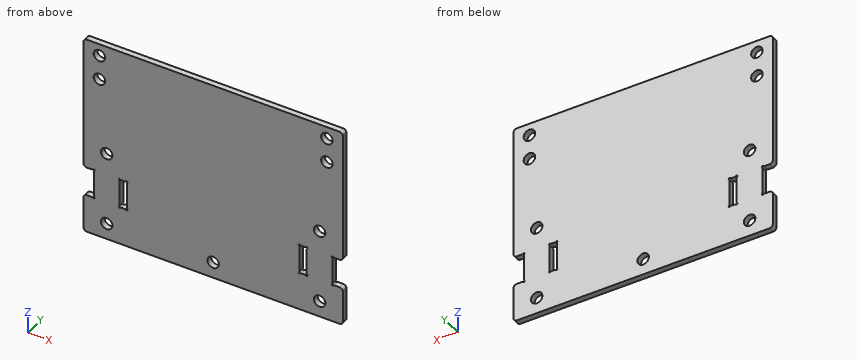
from build123d import *

# Parameters (mm, degrees)
STOCK_BEE_ZERKER_START                     = 4.064
STOCK_BEE_ZERKER_2_0_MULTIBODY_1_OUTLINE_R = 2.2479
STOCK_BEE_ZERKER_2_0_MULTIBODY_1_OUTLINE_W = 2.54
STOCK_BEE_ZERKER_2_0_MULTIBODY_1_OUTLINE_H = 10.89526775
STOCK_BEE_ZERKER_2_0_MULTIBODY_1_DEPTH     = 2.286
SKETCH1_W                                  = 2.794
SKETCH1_H                                  = 11.14926775
SKETCH1_W_2                                = 2.54
SKETCH1_H_2                                = 10.89526775
CUT_EXTRUDE1_DEPTH                         = 67.506087708
SKETCH2_R                                  = 0.3175
CUT_EXTRUDE2_DEPTH                         = 67.327231853
FILLET1_R                                  = 0.635
FILLET2_R                                  = 1.27


# Read off the part's stored shape, not the designer's step: Stock-Bee-zerker 2.0 Multibody-1
with BuildPart() as part:
    # Stock-Bee-zerker 2.0 Multibody-1 outline → Stock-Bee-zerker 2.0 Multibody-1 (new body)
    with BuildSketch(Plane(origin=(0, 0, 0), x_dir=(1, 0, 0), z_dir=(0, 1, 0)).offset(STOCK_BEE_ZERKER_START)):
        Polygon((-50.8, 16.917066125), (-50.8, -35.16122), (50.8, -35.16122), (50.8, 16.917066125), (46.7868, 16.917066125), (46.7868, 27.812333875), (50.8, 27.812333875), (50.8, 42.8625), (-50.8, 42.8625), (-50.8, 27.812333875), (-46.7868, 27.812333875), (-46.7868, 16.917066125), align=None)
        with Locations((-44.45, -30.39872)):
            Circle(STOCK_BEE_ZERKER_2_0_MULTIBODY_1_OUTLINE_R, mode=Mode.SUBTRACT)
        with Locations((-44.45, -20.87372)):
            Circle(STOCK_BEE_ZERKER_2_0_MULTIBODY_1_OUTLINE_R, mode=Mode.SUBTRACT)
        with Locations((44.45, -30.39872)):
            Circle(STOCK_BEE_ZERKER_2_0_MULTIBODY_1_OUTLINE_R, mode=Mode.SUBTRACT)
        with Locations((44.45, -20.87372)):
            Circle(STOCK_BEE_ZERKER_2_0_MULTIBODY_1_OUTLINE_R, mode=Mode.SUBTRACT)
        with Locations((-41.6052, 8.2169)):
            Circle(STOCK_BEE_ZERKER_2_0_MULTIBODY_1_OUTLINE_R, mode=Mode.SUBTRACT)
        with Locations((-35.1536, 22.3647)):
            Rectangle(STOCK_BEE_ZERKER_2_0_MULTIBODY_1_OUTLINE_W, STOCK_BEE_ZERKER_2_0_MULTIBODY_1_OUTLINE_H, mode=Mode.SUBTRACT)
        with Locations((-41.6052, 36.5125)):
            Circle(STOCK_BEE_ZERKER_2_0_MULTIBODY_1_OUTLINE_R, mode=Mode.SUBTRACT)
        with Locations((0, 36.5125)):
            Circle(STOCK_BEE_ZERKER_2_0_MULTIBODY_1_OUTLINE_R, mode=Mode.SUBTRACT)
        with Locations((41.6052, 8.2169)):
            Circle(STOCK_BEE_ZERKER_2_0_MULTIBODY_1_OUTLINE_R, mode=Mode.SUBTRACT)
        with Locations((35.1536, 22.3647)):
            Rectangle(STOCK_BEE_ZERKER_2_0_MULTIBODY_1_OUTLINE_W, STOCK_BEE_ZERKER_2_0_MULTIBODY_1_OUTLINE_H, mode=Mode.SUBTRACT)
        with Locations((41.6052, 36.5125)):
            Circle(STOCK_BEE_ZERKER_2_0_MULTIBODY_1_OUTLINE_R, mode=Mode.SUBTRACT)
    extrude(amount=STOCK_BEE_ZERKER_2_0_MULTIBODY_1_DEPTH)

    # Sketch1 → Cut-Extrude1 (cut, through all)
    # profile 1 of 3: a face of its own
    with BuildSketch(Plane(origin=(0, 6.35, 0), x_dir=(1, 0, 0), z_dir=(0, 1, 0))):
        Polygon((-46.7868, 16.917066125), (-50.8, 16.917066125), (-50.8, -35.16122), (50.8, -35.16122), (50.8, 16.917066125), (46.7868, 16.917066125), (46.7868, 27.812333875), (50.8, 27.812333875), (50.8, 42.8625), (-50.8, 42.8625), (-50.8, 27.812333875), (-46.7868, 27.812333875), align=None)
        Polygon((-46.6598, 16.790066125), (-50.673, 16.790066125), (-50.673, -35.03422), (50.673, -35.03422), (50.673, 16.790066125), (46.6598, 16.790066125), (46.6598, 27.939333875), (50.673, 27.939333875), (50.673, 42.7355), (-50.673, 42.7355), (-50.673, 27.939333875), (-46.6598, 27.939333875), align=None, mode=Mode.SUBTRACT)
    # profile 2 of 3: a face of its own
    with BuildSketch(Plane(origin=(0, 6.35, 0), x_dir=(1, 0, 0), z_dir=(0, 1, 0))):
        with Locations((-35.1536, 22.3647)):
            Rectangle(SKETCH1_W, SKETCH1_H)
        with Locations((-35.1536, 22.3647)):
            Rectangle(SKETCH1_W_2, SKETCH1_H_2, mode=Mode.SUBTRACT)
    # profile 3 of 3: a face of its own
    with BuildSketch(Plane(origin=(0, 6.35, 0), x_dir=(1, 0, 0), z_dir=(0, 1, 0))):
        with Locations((35.1536, 22.3647)):
            Rectangle(SKETCH1_W, SKETCH1_H)
        with Locations((35.1536, 22.3647)):
            Rectangle(SKETCH1_W_2, SKETCH1_H_2, mode=Mode.SUBTRACT)
    extrude(amount=-CUT_EXTRUDE1_DEPTH, mode=Mode.SUBTRACT)

    # Sketch2 → Cut-Extrude2 (cut, through all)
    with BuildSketch(Plane(origin=(0, 6.35, 0), x_dir=(1, 0, 0), z_dir=(0, 1, 0))):
        with Locations((-46.6598, 27.939333875)):
            Circle(SKETCH2_R)
        with Locations((-46.6598, 16.790066125)):
            Circle(SKETCH2_R)
        with Locations((-36.5506, 16.790066125)):
            Circle(SKETCH2_R)
        with Locations((-33.7566, 16.790066125)):
            Circle(SKETCH2_R)
        with Locations((-33.7566, 27.939333875)):
            Circle(SKETCH2_R)
        with Locations((-36.5506, 27.939333875)):
            Circle(SKETCH2_R)
        with Locations((33.7566, 27.939333875)):
            Circle(SKETCH2_R)
        with Locations((36.5506, 27.939333875)):
            Circle(SKETCH2_R)
        with Locations((33.7566, 16.790066125)):
            Circle(SKETCH2_R)
        with Locations((36.5506, 16.790066125)):
            Circle(SKETCH2_R)
        with Locations((46.6598, 16.790066125)):
            Circle(SKETCH2_R)
        with Locations((46.6598, 27.939333875)):
            Circle(SKETCH2_R)
    extrude(amount=-CUT_EXTRUDE2_DEPTH, mode=Mode.SUBTRACT)

    # Fillet1
    fillet1_edges = [part.edges().sort_by_distance(p)[0] for p in [
        (33.7566, 5.207, -17.107566125),
        (33.7566, 5.207, -27.621833875),
        (36.2331, 5.207, -16.790066125),
        (36.5506, 5.207, -27.621833875),
        (-36.5506, 5.207, -17.107566125),
        (-36.5506, 5.207, -27.621833875),
        (-34.0741, 5.207, -16.790066125),
        (-33.7566, 5.207, -27.621833875),
        (-46.6598, 5.207, -27.621833875),
        (-46.6598, 5.207, -17.107566125),
        (46.9773, 5.207, -27.939333875),
        (46.6598, 5.207, -17.107566125),
        (-36.2331, 5.207, -27.939333875),
        (34.0741, 5.207, -27.939333875),
        (36.2331, 5.207, -27.939333875),
        (34.0741, 5.207, -16.790066125),
        (-34.0741, 5.207, -27.939333875),
        (-33.7566, 5.207, -17.107566125),
        (-36.2331, 5.207, -16.790066125),
        (-46.9773, 5.207, -16.790066125),
        (36.5506, 5.207, -17.107566125),
        (46.9773, 5.207, -16.790066125),
        (46.6598, 5.207, -27.621833875),
        (-46.9773, 5.207, -27.939333875),
    ]]
    fillet(fillet1_edges, radius=FILLET1_R)

    # Fillet2
    fillet2_edges = [part.edges().sort_by_distance(p)[0] for p in [
        (-50.673, 5.207, -16.790066125),
        (-50.673, 5.207, 35.03422),
        (50.673, 5.207, 35.03422),
        (50.673, 5.207, -16.790066125),
        (50.673, 5.207, -27.939333875),
        (50.673, 5.207, -42.7355),
        (-50.673, 5.207, -42.7355),
        (-50.673, 5.207, -27.939333875),
    ]]
    fillet(fillet2_edges, radius=FILLET2_R)


solid = part.part
Read the model definition and answer for the solid it produces. Units are mm, in the model's axes. Give positions to 0.01 mm unless a question says otherwise; leave off trailing zeros. Write each loop counter-clockwise with the first axis right and the second up, starting at its lowest first coordinate (ties: lowest second). Pieces come first, ordered by that corner, then holes. Notation, with made-up numbers: M 47,44.5 L 89,44.5 A29 cw 89,82.5 Z; hole C 71,-12 d5. An arc over 180 degrees is marked long. One line per item, written item: value. Start each with the question number.
(1) Find section C-C (y = 5.2). Give the number of separate pieces and of enclosed holes in the cut face, plus the area to 3 significant figures.
(2) Find section B-B (x = 41). Determine the outline of the cut face in (y, z), plus the area to 3 significant figures.
(3) Find the intervals of material crossed by line 1 (Z direction, x = -44.45, y = 5.85); line 2 (X direction, y = 5.3, z = -24); line 3 (X direction, y = 6.1, z = -36.5), in increasing order.
(4) Flat-ended cylindrical pins translate along their axes: pin 1 Ø0.7 at (y, z) = (5.5, -24) entering from +X; pin 2 Ø1.1 at (y, z) = (5, -23.5) entering from -X. Find the tip coordinate at first contact, or state that the pin passes through.
(5) Find section A-A (x = 0). Determine the outline of the cut face in (y, z).
Results below:
1. separate pieces: 1
1. enclosed holes: 11
1. area: 7,580 mm^2
2. outline: M 4.06,-42.74 L 6.35,-42.74 L 6.35,-38.68 L 4.06,-38.68 Z; M 4.06,-34.35 L 6.35,-34.35 L 6.35,-10.38 L 4.06,-10.38 Z; M 4.06,-6.05 L 6.35,-6.05 L 6.35,35.03 L 4.06,35.03 Z
2. area: 158 mm^2
3. line 1: z = -42.74 to 18.63, 23.12 to 28.15, 32.65 to 35.03
3. line 2: x = -46.66 to -36.55, -33.76 to 33.76, 36.55 to 46.66
3. line 3: x = -50.67 to -43.85, -39.36 to -2.25, 2.25 to 39.36, 43.85 to 50.67
4. pin 1: stops at x = 46.66
4. pin 2: stops at x = -46.66
5. outline: M 4.06,-42.74 L 6.35,-42.74 L 6.35,-38.76 L 4.06,-38.76 Z; M 4.06,-34.26 L 6.35,-34.26 L 6.35,35.03 L 4.06,35.03 Z
